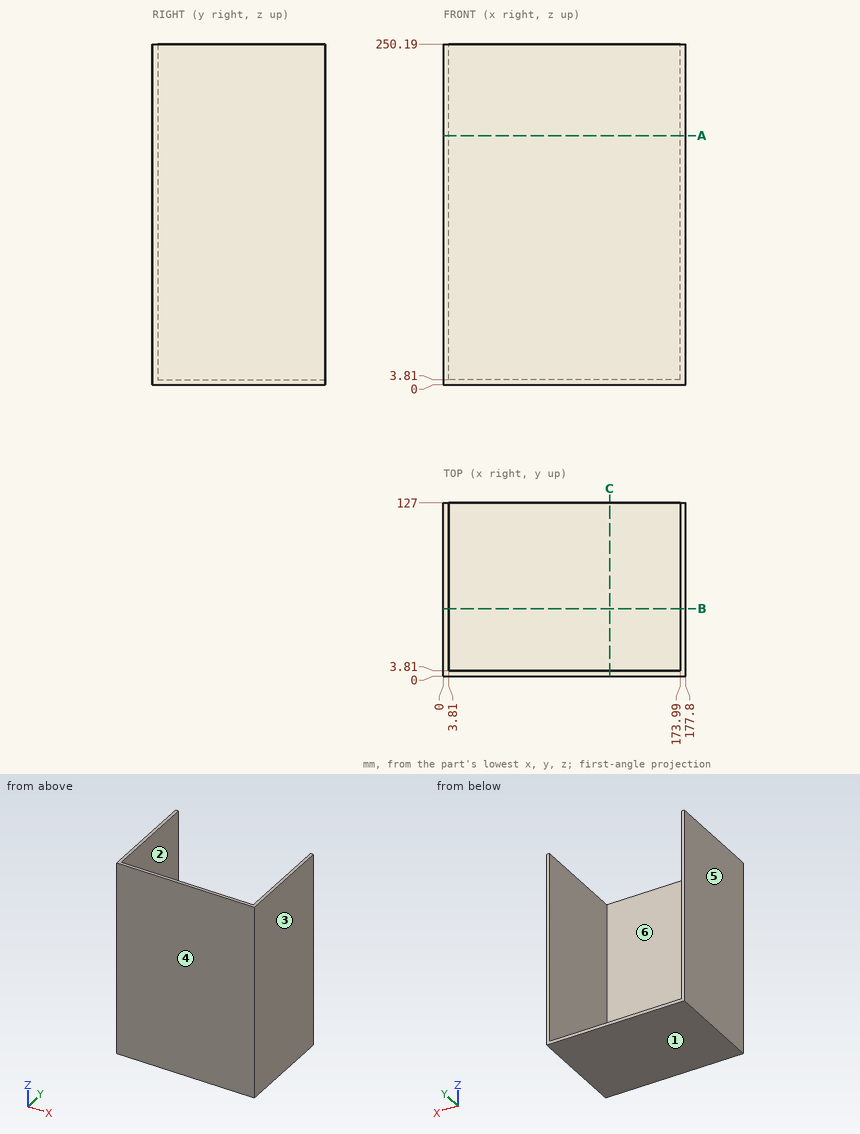
For this review, use the dimensioned drawing (mm, ordinates from the lowest corner) and the shaded views. A direction names the side the tool comes from. Give positions to 0.01 mm unless a question says otherwise; leave off trailing zeros. Write each loop counter-clockwise with the first axis right and the second up, starting at its lowest first coordinate (ties: lowest second). Pieces come first, ordered by that corner, then holes.
(1) Consider section A-A, the plane z = 183. Give the boundary of the cut face in (x, y).
(2) The part is to be moulded in two halves that separate along X. For the marked faces 3, 4, 5 and 6, say which applies: released by +X, released by -X, zero draft, split by the parting line, or undercut.
(3) Tool access review of the marked faces 1 and 2: name each direction out of +Z, -Z, +X, -X, +Y, -Y from which nothing blocks a thin tool from reaching the whole face with its end or side.
(4) For P1, Ø3, axis at x = 121, y = 13.5, coming from the -Z side; P2, Ø2, axis at x = 48, y = 34, coming from the +Z side; P3, Ø10, axis at x = 73, z = 199.5, coming from the +Y side, all flat-tipped, find the tip position at first contact; note any pin that passes through.
(5) Consider section B-B, the plane y = 49.5. Give the boundary of the cut face in (x, z).
(6) To check wall thickness, follow L1, parallel to X at y = 47.5, z = 161.5; L2, parallel to Z at x = 86.5, y = 116.5. State the ranges of each line that lie inside material, in increasing order.
(7) Consider section C-C, the plane x = 122. Give the boundary of the cut face in (y, z).
Returned:
1. outline: (0, 0) - (177.8, 0) - (177.8, 127) - (173.99, 127) - (173.99, 3.81) - (3.81, 3.81) - (3.81, 127) - (0, 127) - close
2. face 3: released by +X
2. face 4: zero draft
2. face 5: released by -X
2. face 6: undercut
3. face 1: -Z, +X, -X, +Y, -Y
3. face 2: +Z, +Y
4. P1: stops at z = 0
4. P2: stops at z = 3.81
4. P3: stops at y = 3.81
5. outline: (0, 0) - (177.8, 0) - (177.8, 250.19) - (173.99, 250.19) - (173.99, 3.81) - (3.81, 3.81) - (3.81, 250.19) - (0, 250.19) - close
6. L1: x = 0 to 3.81, 173.99 to 177.8
6. L2: z = 0 to 3.81
7. outline: (0, 0) - (127, 0) - (127, 3.81) - (3.81, 3.81) - (3.81, 250.19) - (0, 250.19) - close
